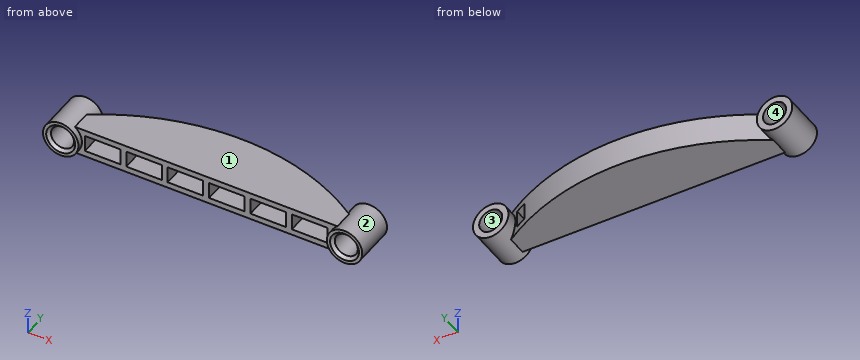
from build123d import *

# Parameters (mm, degrees)
EXTRUDE_2_DEPTH              = 12
EXTRUDE_3_DEPTH              = 5
EXTRUDE_3_DEPTH_BACK         = 30
SKETCH_4_R                   = 15
CUT_EXTRUDE_2_REACH          = 146.741
CUT_EXTRUDE_2_END_RADIUS     = 195
SKETCH_5_W                   = 30
SKETCH_5_H                   = 14
PATTERN_LINEAR_1_COUNT       = 6
PATTERN_LINEAR_1_PITCH       = 35
HOLE_WIZARD_M221_D           = 19.5
HOLE_WIZARD_M221_CSINK_D     = 24.5
HOLE_WIZARD_M221_CSINK_ANGLE = 90


with BuildPart() as part:
    # Эскиз2 → Бобышка-Вытянуть2 (new, symmetric)
    with BuildSketch(Plane.XY):
        with BuildLine():
            Line((120, 0), (-120, 0))
            Line((-120, 0), (-120, 10))
            ThreePointArc((-120, 10), (0, 50), (120, 10))
            Line((120, 10), (120, 0))
        make_face()
    extrude(amount=EXTRUDE_2_DEPTH, both=True)

    # Эскиз4 → Бобышка-Вытянуть3 (add, two sides: drawn at the far end of the back side and taken through both)
    with BuildSketch(Plane.XZ.offset(-EXTRUDE_3_DEPTH_BACK)):
        with Locations((-120, 0)):
            Circle(SKETCH_4_R)
        with Locations(Location((120, 0, 0), (0, 0, 180))):
            Circle(SKETCH_4_R)
    extrude(amount=EXTRUDE_3_DEPTH + EXTRUDE_3_DEPTH_BACK)

    # Вырез-Вытянуть2: up to this cylinder (the profile starts inside it)
    cut_extrude_2_end = Plane(origin=(0, -150, 0), z_dir=(0, 0, -1)) * Cylinder(CUT_EXTRUDE_2_END_RADIUS, 684.482, mode=Mode.PRIVATE)
    # Эскиз5 → Вырез-Вытянуть2 (cut, up to the surface)
    with BuildSketch(Plane.XZ, mode=Mode.PRIVATE) as cut_extrude_2_sk1:
        with Locations((-87.5, 0)):
            Rectangle(SKETCH_5_W, SKETCH_5_H)
    cut_extrude_2_tool1 = extrude(cut_extrude_2_sk1.sketch, amount=-CUT_EXTRUDE_2_REACH, mode=Mode.PRIVATE) & cut_extrude_2_end
    cut_extrude_2 = cut_extrude_2_tool1.solids().sort_by_distance((-87.5, 0, 0))[0]
    add(cut_extrude_2, mode=Mode.SUBTRACT)

    # Линейный массив1: Вырез-Вытянуть2 ×6
    with Locations(*[(i * PATTERN_LINEAR_1_PITCH, 0, 0) for i in range(1, PATTERN_LINEAR_1_COUNT)]):
        add(cut_extrude_2, mode=Mode.SUBTRACT)

    # Отверстие обработанное метчиком M221 (through all)
    with Locations(Plane(origin=(0, -5, 0), x_dir=(-1, 0, 0), z_dir=(0, -1, 0))):
        with Locations((-120, 0), (120, 0)):
            CounterSinkHole(HOLE_WIZARD_M221_D / 2, HOLE_WIZARD_M221_CSINK_D / 2, counter_sink_angle=HOLE_WIZARD_M221_CSINK_ANGLE)


solid = part.part
Design review of the part built by this model. Coordinates are the model's own, in mm. Face numbers are marked on the shaded views. Round coordinates to 2 decimals unless told otherwise and drop trailing zeros. Loops run counter-clockwise (first coordinate to the right, second up) from the corner with the lowest first, then second, coordinate; pieces in that order, holes last. Notation, with made-up numbers: (89.25, -4.75) - (94.25, -4.75) arc R25 cw to (94.25, 34.25) - close; hole circle Ø7 at (77, -3.75). An arc over 180 degrees is marked (long way). One line per item, written item: value. Start each with the question number.
1) Consider section A-A on x = -120. Give the boundary of the cut face in (y, z).
2) Insertion check: pin 1 Ø6 at (x, z) = (-11, 1) entering from -Y; pin 2 Ø15 at (x, y) = (19, 15) entering from -Z; pin 3 Ø11 at (y, z) = (17, -2) entering from -X; pin 4 Ø4 at (x, y) = (15, 33) entering from +Z. Each pin has a flat end and moves straight along its axis. Give the tip position at first contact, or say it passes through.
3) Draft analysis for pull direction Z (two halves, no side actions). For the marked faces 1, 2, 3 and 4, state which applies: +Z half, -Z half, draft (parallel to the pull), parting line (faces both ways), or undercut.
4) Consider section B-B on y = 9. Give the number of separate pieces and of enclosed holes in the cut face, then the cut area to 3 significant figures.
5) To check wall thickness, follow L1, parallel to Z at x = -81.5, y = 25; L2, parallel to X at y = 17, z = 7.5; L3, parallel to X at y = 21, z = 11. State the ranges of each line that lie inside material, in increasing order. Write a range as from..to.
6) Consider section D-D on x = 17. Give the boundary of the cut face in (y, z).
Reported:
1. outline: (-5, -15) - (30, -15) - (30, -9.75) - (-2.5, -9.75) - (-5, -12.25) - close; (-5, 12.25) - (-2.5, 9.75) - (30, 9.75) - (30, 15) - (-5, 15) - close
2. pin 1: stops at y = 25.98
2. pin 2: stops at z = -12
2. pin 3: stops at x = -135
2. pin 4: stops at z = 12
3. face 1: +Z half
3. face 2: parting line
3. face 3: undercut
3. face 4: undercut
4. separate pieces: 1
4. enclosed holes: 8
4. area: 3,420 mm^2
5. L1: z = -12..-7, 7..12
5. L2: x = -132.99..-126.23, -113.77..113.77, 126.23..132.99
5. L3: x = -130.2..-109.8, -103.73..103.73, 109.8..130.2
6. outline: (0, -12) - (49.28, -12) - (49.28, 12) - (0, 12) - (0, 7) - (24.01, 7) - (24.01, -7) - (0, -7) - close
